Drawing for the job (mm, zero at the part's lowest x, y, z). Coordinates: 2 decimals unless noted, no trailing zeros. Write each loop counter-clockwise with the first axis right and the second up, starting at its lowest first coordinate (ties: lowest second). Pieces come first, ordered by that corner, then holes. Notation, with made-up numbers: M 70.25,50 L 81.25,50 A21 ccw 81.25,70 Z; hole C -30.5,38 d4. An arc over 180 degrees is marked long. Use a Markdown table: item, result. Add a question column.
Q1. Mould opens along X. For the marked faces 1 and 2 say: released by +X, released by -X, zero draft, split by the parting line, or undercut.
Q2. Slice it at C-C on y = 20.5. Write the cut outline in (x, z).
Q3. Wall check: L1, parallel to Y at x = 13.25, z = 16; L2, parallel to Z at x = 11.5, y = 15.5; L3, parallel to X at y = 20, z = 2. Give the ranges that are in metal, low to high. Write a range as from..to.
Q4. Slice it at B-B on z = 11.25. Write the cut outline in (x, y), then the cut area to 3 significant figures.
Q5. Pin check, flat tips, straight feed: pin 1 Ø12 at (x, y) = (4.5, 13.5) entering from -Z (3 decimals); pin 2 Ø0.8 at (x, y) = (15.5, 3) entering from -Z; pin 3 Ø1.2 at (x, y) = (7, 3) entering from +Z. Stop position of each tip, or through.
Q6. Slice it at A-A on x = 11.25. Write the cut outline in (y, z), then the cut area to 3 significant figures.
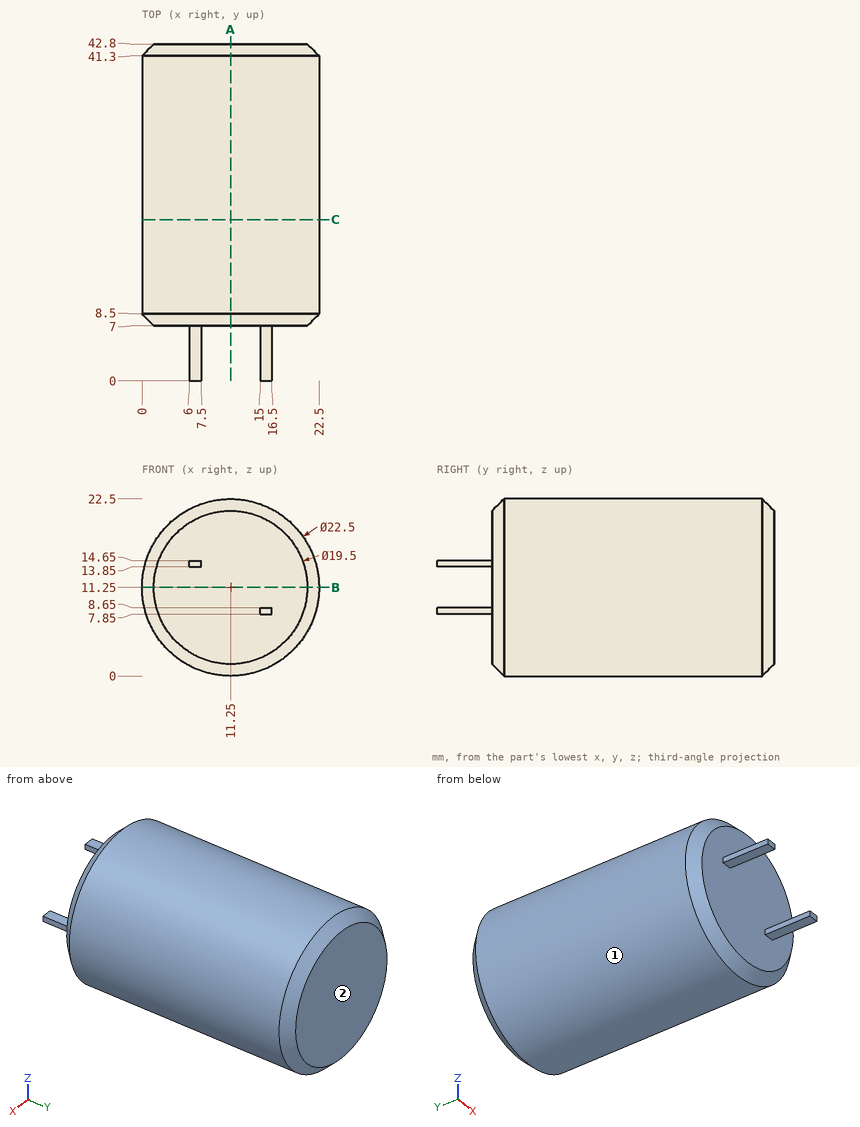
Recorded:
| question | item | result |
|---|---|---|
| 1 | face 1 | split by the parting line |
| 1 | face 2 | zero draft |
| 2 | outline | C 11.25,11.25 d22.5 |
| 3 | L1 | 7..42.8 |
| 3 | L2 | 0..22.5 |
| 3 | L3 | 4.85..17.65 |
| 4 | outline | M 0,8.5 L 1.5,7 L 21,7 L 22.5,8.5 L 22.5,41.3 L 21,42.8 L 1.5,42.8 L 0,41.3 Z |
| 4 | area | 801 mm² |
| 5 | pin 1 | z = 0.025 |
| 5 | pin 2 | z = 7.85 |
| 5 | pin 3 | z = 14.65 |
| 6 | outline | M 7,1.5 L 8.5,0 L 41.3,0 L 42.8,1.5 L 42.8,21 L 41.3,22.5 L 8.5,22.5 L 7,21 Z |
| 6 | area | 801 mm² |
